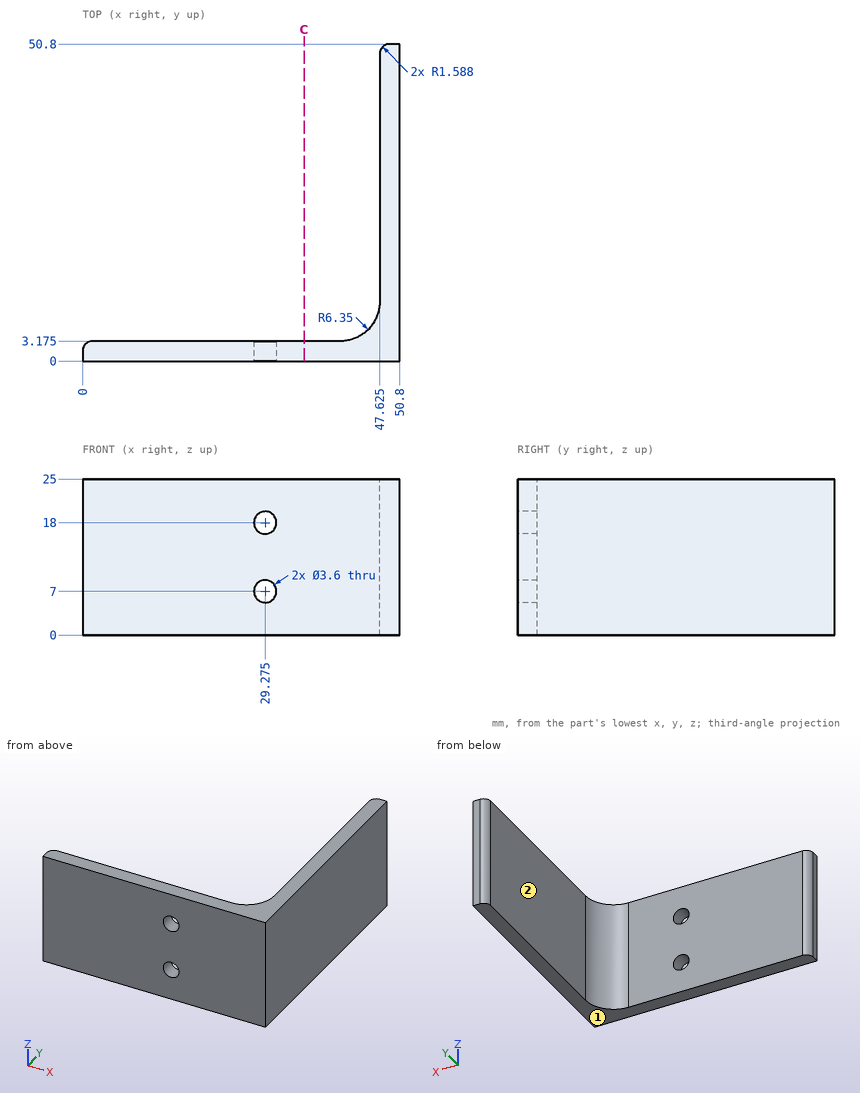
Here's the drawing with two shaded views (mm, measured from the low corner). I have some questions. A direction names the side the tool comes from. Round coordinates to 2 decimals unless told otherwise and drop trailing zeros. Order: outer loops, then holes, each group sorted by start corner. A loop starts at its lowest first (then second) coordinate and runs counter-clockwise, first axis right, second up. Notation, with made-up numbers: (30, 68) -> (37, 68) arc R19 cw to (37, 75) -> close; hole circle Ø7 at (79.5, 22). An arc over 180 degrees is marked (long way). Use a Markdown table: item, result. Add a question column.
(1) Suppose I cut it at C-C, the plane x = 35.5. Please give me the cut outline in (y, z) (1 decimal).
(2) I need wall thicknesses on line 1 along X through (y, z) = (1.1, 7) (1 decimal); line 2 along X through (y, z) = (40.5, 18.25) (1 decimal); line 3 along Y through (x, z) = (15, 20.75) (1 decimal). Which ranges of each line are inside material? Lowest first, please.
(3) For pin 1 Ø8 at (y, z) = (12.5, 6.5) entering from -X; pin 2 Ø6 at (y, z) = (9.5, 8) entering from -X; pin 3 Ø7.5 at (y, z) = (25, 10) entering from -X (1 decimal), each with a flat end and sliding along its axis, tell me the tip position at first contact or that it passes through.
(4) For the marked faces 1 and 2, which set-ups out of +Z, -Z, +X, -X, +Y, -Y let a thin tool reach every point of the face, with its end or its side?
Verdict:
| question | item | result |
|---|---|---|
| 1 | outline | (0, 0) -> (3.2, 0) -> (3.2, 25) -> (0, 25) -> close |
| 2 | line 1 | 0 to 27.5, 31.1 to 50.8 |
| 2 | line 2 | 47.6 to 50.8 |
| 2 | line 3 | 0 to 3.2 |
| 3 | pin 1 | x = 47.54 |
| 3 | pin 2 | x = 46.86 |
| 3 | pin 3 | x = 47.6 |
| 4 | face 1 | -Z, +X, -X, +Y, -Y |
| 4 | face 2 | +Z, -Z, -X, +Y |
